```python
from build123d import *

# Parameters (mm, degrees)
F1_DEPTH       = 63.5
F2_R           = 19.05
F3_DEPTH       = 9.525
F4_R           = 21.59
F4_R_2         = 19.05
F5_DEPTH       = 6.35
F6_R           = 2.53999
F8_D           = 6.35
F8_CSINK_D     = 19.05
F8_CSINK_ANGLE = 82


# Not quite as in the source:
# - a fillet or chamfer is up to 0.001 mm smaller than in the source, because OpenCascade refuses the exact size


with BuildPart() as f1:
    # F0 (on Right) → F1 (new body)
    with BuildSketch(Plane.YZ):
        Polygon((0, 21.59), (0, 0), (95.25, 0), (95.25, 46.99), (44.45, 46.99), (44.45, 21.59), align=None)
    extrude(amount=-F1_DEPTH)

    # F2 (on face) → F3 (cut)
    with BuildSketch(Plane.XY.offset(21.59)):
        with Locations((-31.75, 22.225)):
            Circle(F2_R)
    extrude(amount=-F3_DEPTH, mode=Mode.SUBTRACT)

    # F4 (on face) → F5 (join)
    with BuildSketch(Plane.XY.offset(21.59)):
        with Locations((-31.75, 22.225)):
            Circle(F4_R)
        with Locations((-31.75, 22.225)):
            Circle(F4_R_2, mode=Mode.SUBTRACT)
    extrude(amount=F5_DEPTH)

    # F6 (radius 2.54 in the source; OpenCascade refuses exactly that, so slightly less here)
    f6_edges = [f1.edges().sort_by_distance(p)[0] for p in [
        (-53.34, 22.225, 27.94),
    ]]
    fillet(f6_edges, radius=F6_R)

    # F8 (through all)
    with Locations(Plane.XY.offset(46.99)):
        with Locations((-50.8, 82.55), (-12.7, 82.55)):
            CounterSinkHole(F8_D / 2, F8_CSINK_D / 2, counter_sink_angle=F8_CSINK_ANGLE)


solid = f1.part
```
Design review of the part built by this model. Coordinates are the model's own, in mm. A direction names the side the tool comes from. Round coordinates to 2 decimals unless told otherwise and drop trailing zeros. Write each loop counter-clockwise with the first axis right and the second up, starting at its lowest first coordinate (ties: lowest second). Pieces come first, ordered by that corner, then holes.
Item 1: The part is to be moulded in two halves that separate along Y. For faces 1 (the flat face through (0, 58, 19)), 2 (the flat face through (-31, 95.25, 23)), 3 (the cylindrical face through (-12.01, 79.45, 19.56)), say which applies: +Y half, -Y half, draft (parallel to the pull), parting line (faces both ways), or undercut.
Item 2: We need section A-A on y = 82.55. Write out the cut boundary in (x, z) (3 decimals), and give its area (3 significant figures).
Item 3: We need section D-D on z = 30. Write out the cut boundary in (x, y) (3 decimals), and give its area (3 significant figures).
Item 4: For faces 4 (the flat face through (-63.5, 58, 19)), 5 (the flat face through (-31, 44.45, 34)), 6 (the flat face through (-32, 22, 12.065)), list the 3-axis set-ups (+Z, -Z, +X, -X, +Y, -Y) from which the entire face can be reached by the end or side of a thin tool; tool diameter is ignored.
Item 5: We need section C-C on z = 19.5. Write out the cut boundary in (x, y) (3 decimals).
Item 6: Clearance check with flat-ended pins moving along their axes: pin 1 Ø5 at (x, y) = (-12.7, 82.55) entering from -Z; pin 2 Ø1 at (y, z) = (18.5, 27) entering from -X; pin 3 Ø22 at (x, y) = (-31.5, 27) entering from +Z (3 decimals). State where each tip first meets the part, or that it passes through.
Item 7: For probe 1 along X at (y, z) = (82.55, 21) (3 decimals); probe 2 along Y at (x, z) = (-50.8, 30) (3 decimals); probe 3 along X at (y, z) = (82, 12), list the stretches that pass through material, from the lowest coordinate up.
Returned:
1. face 1: draft
1. face 2: +Y half
1. face 3: undercut
2. outline: (-63.5, 0) - (-53.975, 0) - (-53.975, 39.685) - (-60.325, 46.99) - (-63.5, 46.99) - close; (-47.625, 0) - (-15.875, 0) - (-15.875, 39.685) - (-22.225, 46.99) - (-41.275, 46.99) - (-47.625, 39.685) - close; (-9.525, 0) - (0, 0) - (0, 46.99) - (-3.175, 46.99) - (-9.525, 39.685) - close
2. area: 2,290 mm2
3. outline: (-63.5, 44.45) - (0, 44.45) - (0, 95.25) - (-63.5, 95.25) - close; hole circle Ø6.35 at (-50.8, 82.55); hole circle Ø6.35 at (-12.7, 82.55)
3. area: 3,160 mm2
4. face 4: +Z, -Z, -X, +Y, -Y
4. face 5: +Z, +X, -X
4. face 6: +Z
5. outline: (-63.5, 0) - (0, 0) - (0, 95.25) - (-63.5, 95.25) - close; hole circle Ø6.35 at (-50.8, 82.55); hole circle Ø38.1 at (-31.75, 22.225); hole circle Ø6.35 at (-12.7, 82.55)
6. pin 1: passes through
6. pin 2: stops at x = -52.78
6. pin 3: stops at z = 12.065
7. probe 1: x = -63.5 to -53.975, -47.625 to -15.875, -9.525 to 0
7. probe 2: y = 44.45 to 79.375, 85.725 to 95.25
7. probe 3: x = -63.5 to -53.93, -47.67 to -15.83, -9.57 to 0
